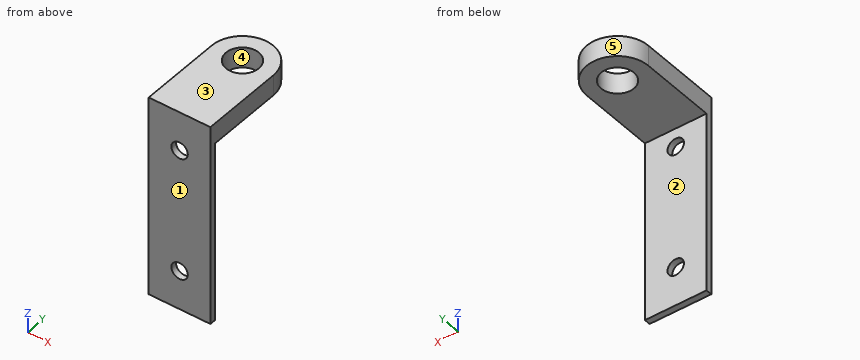
Autodesk Inventor part; units mm, degrees
ref_plane "YZ Plane" through (0, 0, 0) normal (1, 0, 0) x (0, 1, 0)
ref_plane "XZ Plane" through (0, 0, 0) normal (0, 1, 0) x (-1, 0, 0)
ref_plane "XY Plane" through (0, 0, 0) normal (0, 0, 1) x (1, 0, 0)
sketch "Sketch1" plane through (0, 0, 0) normal (0, 0, 1) x (1, 0, 0)
  circle A0 centre (0, 0) radius 4
  arc A1 (7.5, 0) -> (-7.5, 0) centre (0, 0) ccw
  line L0 (-7.5, 0) -> (7.5, 0)
  line L1 (7.5, 0) -> (7.5, -20)
  line L2 (7.5, -20) -> (-7.5, -20)
  line L3 (-7.5, -20) -> (-7.5, 0)
  dimension "d0" = 8
  dimension "d1" = 15
  dimension "d2" = 15
  dimension "d3" = 20
extrude "Extrusion1" add sketch "Sketch1" along normal mid plane 5 contours L0 L1 L2 L3 A0 | A0 L0 A1
sketch "Sketch2" plane through (0, 0, -2.5) normal (0, 0, -1) x (-1, 0, 0)
  line L0 (7.5, -20) -> (-7.5, -20)
  line L1 (-7.5, -20) -> (7.5, -20)
  line L2 (7.5, -20) -> (7.5, -18.5)
  line L3 (7.5, -18.5) -> (-7.5, -18.5)
  line L4 (-7.5, -18.5) -> (-7.5, -20)
  point P0 (0, 0)
  dimension "d6" = 15
  dimension "d7" = 1.5
extrude "Extrusion2" add sketch "Sketch2" along normal blind 44
sketch "Sketch3" plane through (-7.5, -18.5, -2.5) normal (0, 1, 0) x (1, 0, 0)
  line L0 (0, -5) -> (15, -5)
  line L1 (7.5, -5) -> (7.5, 4.5)
  line L2 (7.5, 4.5) -> (7.5, 34.5)
  point P0 (7.5, -2.5)
  dimension "d10" = 9.5
  dimension "d11" = 30
hole "Hole1" at (0, -18.5, -7) at (0, -18.5, -37) direction (0, -1, 0) diameter 4 depth 6
properties part number "Half Bearing Block"
The model under review builds one solid part; all positions refer to its coordinate system, in mm. Face numbers are marked on the shaded views. A direction names the side the tool comes from. Give positions to 0.01 mm unless a question says otherwise; leave off trailing zeros. Write each loop counter-clockwise with the first axis right and the second up, starting at its lowest first coordinate (ties: lowest second). Pieces come first, ordered by that corner, then holes.
1. Add section B-B, the plane z = -7. Write out the cut boundary in (x, y), plus the area to 3 significant figures.
2. Add section D-D, the plane x = 4.5. Write out the cut boundary in (y, z), plus the area to 3 significant figures.
3. Draft analysis for pull direction X (two halves, no side actions). For the marked faces 3, 4 and 5, state which applies: +X half, -X half, draft (parallel to the pull), parting line (faces both ways), or undercut.
4. Add section C-C, the plane y = 2.5. Write out the cut boundary in (x, z).
5. For P1, Ø4.5, axis at x = 0, z = -7, coming from the +Y side, flat-tipped, find the tip position at first contact; note if it passes through.
6. Add section A-A, the plane x = 0. Write out the cut boundary in (y, z).
7. Tool access review of the marked faces 1 and 2: name each direction out of +Z, -Z, +X, -X, +Y, -Y from which nothing blocks a thin tool from reaching the whole face with its end or side.
8. Wall thickness on L1, parallel to Z at x = 0, y = -19.05; L2, parallel to X at y = 0, z = -1.4; L3, parallel to Y at x = 4, z = -29: over which ranges is each line inside the solid? List them lowest first.
Worked answers:
1. outline: (-7.5, -20) - (-2, -20) - (-2, -18.5) - (-7.5, -18.5) - close; (2, -20) - (7.5, -20) - (7.5, -18.5) - (2, -18.5) - close
1. area: 16.5 mm2
2. outline: (-20, -46.5) - (-18.5, -46.5) - (-18.5, -2.5) - (6, -2.5) - (6, 2.5) - (-20, 2.5) - close
2. area: 196 mm2
3. face 3: draft
3. face 4: undercut
3. face 5: parting line
4. outline: (-7.07, -2.5) - (-3.12, -2.5) - (-3.12, 2.5) - (-7.07, 2.5) - close; (3.12, -2.5) - (7.07, -2.5) - (7.07, 2.5) - (3.12, 2.5) - close
5. P1: stops at y = -18.5
6. outline: (-20, -46.5) - (-18.5, -46.5) - (-18.5, -39) - (-20, -39) - close; (-20, -35) - (-18.5, -35) - (-18.5, -9) - (-20, -9) - close; (-20, -5) - (-18.5, -5) - (-18.5, -2.5) - (-4, -2.5) - (-4, 2.5) - (-20, 2.5) - close; (4, -2.5) - (7.5, -2.5) - (7.5, 2.5) - (4, 2.5) - close
7. face 1: +Z, -Z, +X, -X, -Y
7. face 2: -Z, +X, -X, +Y
8. L1: z = -46.5 to -39, -35 to -9, -5 to 2.5
8. L2: x = -7.5 to -4, 4 to 7.5
8. L3: y = -20 to -18.5
